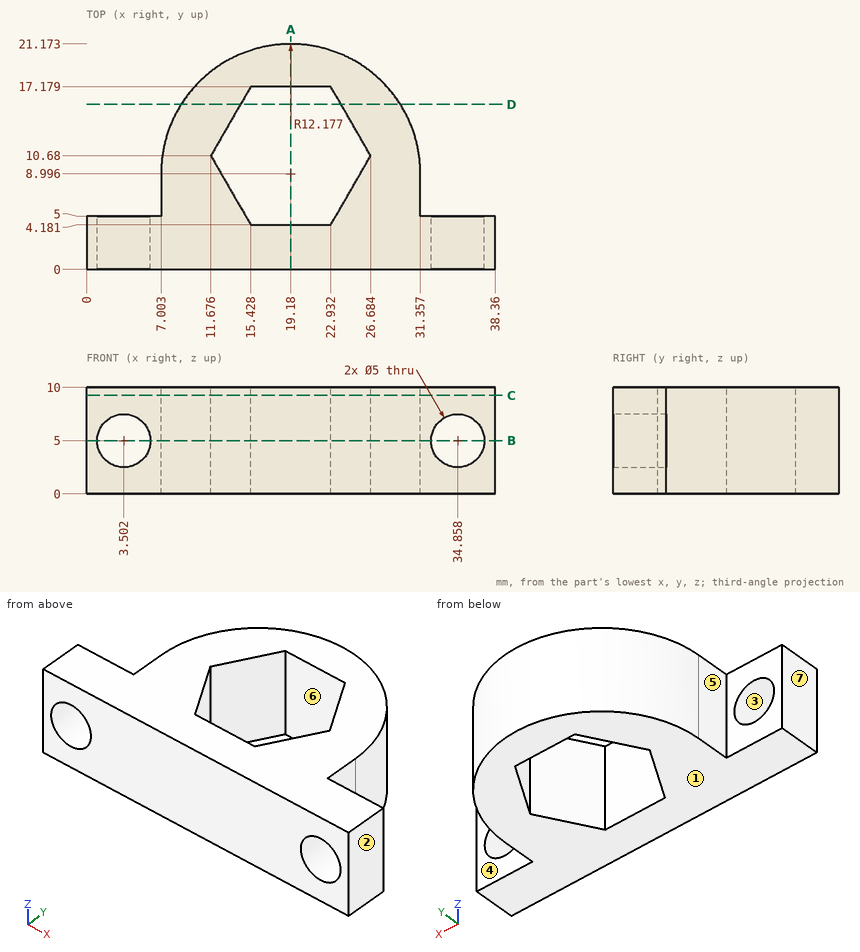
The figure shows three views and two pictorial views of one solid part (mm, origin at its lowest corner). Answer the questions. A direction names the side the tool comes from. Give positions to 0.01 mm unless a question says otherwise; leave off trailing zeros. Write each loop counter-clockwise with the first axis right and the second up, starting at its lowest first coordinate (ties: lowest second). Pieces come first, ordered by that corner, then holes. Notation, with made-up numbers: M -26.75,28 L 4.25,28 A33 ccw 4.25,58 Z; hole C 10,35 d10. An arc over 180 degrees is marked long. One line per item, written item: value. Start each with the question number.
(1) Find section A-A (x = 19.18). Determine the outline of the cut face in (y, z).
(2) Determine the mould class of the marked faces 1, 2 and 3 for opening direction Z: pulls with the +Z half, pulls with the -Z half, needs draft (parallel to the pull), parting line crosses it, or undercut.
(3) Find section C-C (z = 9.25). Determine the outline of the cut face in (x, y) (1 decimal).
(4) Flat-ended cylindrical pins translate along their axes: pin 1 Ø4 at (x, z) = (28, 4) entering from +Y (1 decimal); pin 2 Ø4.5 at (y, z) = (7.5, 3) entering from -X; pin 3 Ø2 at (x, z) = (5, 3.5) entering from +Y; pin 4 Ø4 at (x, z) = (3.5, 5) entering from +Y. Find the tip coordinate at first contact, or state that the pin passes through.
(5) Find section B-B (z = 5). Determine the outline of the cut face in (x, y) (1 decimal).
(6) A tool of negligible diameter and unlimited length cuts with its end or side. For the marked faces 4, 5, 6 and 7, from which of +Z, -Z, +X, -X, +Y, -Y can it reach the whole face along a straight path? Write none if from no direction.
(7) Find the intervals of material crossed by line 1 (X direction, y = 2.95, z = 5); line 2 (X direction, y = 3.25, z = 5.25) (1 decimal); line 3 (X direction, y = 4.25, z = 5), in increasing order.
(8) Find section D-D (y = 15.5). Determine the outline of the cut face in (x, z) (1 decimal).
Results below:
1. outline: M 0,0 L 4.18,0 L 4.18,10 L 0,10 Z; M 17.18,0 L 21.17,0 L 21.17,10 L 17.18,10 Z
2. face 1: pulls with the -Z half
2. face 2: needs draft
2. face 3: undercut
3. outline: M 0,0 L 38.4,0 L 38.4,5 L 31.4,5 L 31.4,9 A12.2 ccw 7,9 L 7,5 L 0,5 Z; hole M 11.7,10.7 L 15.4,4.2 L 22.9,4.2 L 26.7,10.7 L 22.9,17.2 L 15.4,17.2 Z
4. pin 1: stops at y = 19.1
4. pin 2: stops at x = 7
4. pin 3: stops at y = 5
4. pin 4: passes through
5. outline: M 0,0 L 1,0 L 1,5 L 0,5 Z; M 6,0 L 32.4,0 L 32.4,5 L 31.4,5 L 31.4,9 A12.2 ccw 7,9 L 7,5 L 6,5 Z; M 37.4,0 L 38.4,0 L 38.4,5 L 37.4,5 Z; hole M 11.7,10.7 L 15.4,4.2 L 22.9,4.2 L 26.7,10.7 L 22.9,17.2 L 15.4,17.2 Z
6. face 4: +Z, -Z, +X, +Y
6. face 5: +Z, -Z, -X, +Y
6. face 6: +Z, -Z
6. face 7: +Z, -Z, -X, +Y, -Y
7. line 1: x = 0 to 1, 6 to 32.36, 37.36 to 38.36
7. line 2: x = 0 to 1, 6 to 32.4, 37.3 to 38.4
7. line 3: x = 0 to 1, 6 to 15.39, 22.97 to 32.36, 37.36 to 38.36
8. outline: M 8.9,0 L 14.5,0 L 14.5,10 L 8.9,10 Z; M 23.9,0 L 29.5,0 L 29.5,10 L 23.9,10 Z
